```python
from build123d import *

# Parameters (mm, degrees)
SKETCH1_R           = 11.15
BOSS_EXTRUDE1_DEPTH = 50
SKETCH2_R           = 7.75
BOSS_EXTRUDE2_DEPTH = 8
SKETCH3_R           = 5.825
BOSS_EXTRUDE3_DEPTH = 10
SKETCH4_R           = 9.1
CUT_EXTRUDE1_DEPTH  = 35
SKETCH5_R           = 2.75
CUT_EXTRUDE2_DEPTH  = 70.804333676
SKETCH10_W          = 3
SKETCH10_H          = 11.4427922
BOSS_EXTRUDE5_DEPTH = 6
SKETCH12_W          = 6
SKETCH12_H          = 1
CUT_EXTRUDE6_DEPTH  = 6
CUT_EXTRUDE8_DEPTH  = 18
SKETCH14_W          = 6
SKETCH14_H          = 10.4427922
CUT_EXTRUDE9_DEPTH  = 8


with BuildPart() as part:
    # Sketch1 → Boss-Extrude1 (new body)
    with BuildSketch(Plane(origin=(0, 0, 0), x_dir=(1, 0, 0), z_dir=(0, 1, 0))):
        with Locations(Location((0, 0, 0), (0, 0, 270))):
            Circle(SKETCH1_R)
    extrude(amount=BOSS_EXTRUDE1_DEPTH)

    # Sketch2 → Boss-Extrude2 (add)
    with BuildSketch(Plane(origin=(0, 50, 0), x_dir=(1, 0, 0), z_dir=(0, 1, 0))):
        with Locations(Location((0, 0, 0), (0, 0, 270))):
            Circle(SKETCH2_R)
    extrude(amount=BOSS_EXTRUDE2_DEPTH)

    # Sketch3 → Boss-Extrude3 (add)
    with BuildSketch(Plane(origin=(0, 58, 0), x_dir=(1, 0, 0), z_dir=(0, 1, 0))):
        with Locations(Location((0, 0, 0), (0, 0, 270))):
            Circle(SKETCH3_R)
    extrude(amount=BOSS_EXTRUDE3_DEPTH)

    # Sketch4 → Cut-Extrude1 (cut)
    with BuildSketch(Plane.XZ):
        with Locations(Location((0, 0, 0), (0, 0, 270))):
            Circle(SKETCH4_R)
    extrude(amount=-CUT_EXTRUDE1_DEPTH, mode=Mode.SUBTRACT)

    # Sketch5 → Cut-Extrude2 (cut, through all)
    with BuildSketch(Plane(origin=(0, 68, 0), x_dir=(1, 0, 0), z_dir=(0, 1, 0))):
        with Locations(Location((0, 0, 0), (0, 0, 270))):
            Circle(SKETCH5_R)
    extrude(amount=-CUT_EXTRUDE2_DEPTH, mode=Mode.SUBTRACT)


with BuildPart() as body_2:
    # Sketch10 → Boss-Extrude5 (new body)
    with BuildSketch(Plane(origin=(0, 58, 0), x_dir=(1, 0, 0), z_dir=(0, 1, 0))):
        with Locations((-1.5, -13.4713961)):
            Rectangle(SKETCH10_W, SKETCH10_H)
        with Locations((1.5, -13.4713961)):
            Rectangle(SKETCH10_W, SKETCH10_H)
    extrude(amount=-BOSS_EXTRUDE5_DEPTH)

    # Sketch12 → Cut-Extrude6 (cut)
    with BuildSketch(Plane(origin=(0, 58, 0), x_dir=(1, 0, 0), z_dir=(0, 1, 0))):
        with Locations((0, -8.25)):
            Rectangle(SKETCH12_W, SKETCH12_H)
    extrude(amount=-CUT_EXTRUDE6_DEPTH, mode=Mode.SUBTRACT)


with BuildPart() as cut_extrude8_tool:
    # Sketch11 → Cut-Extrude8 (new body)
    with BuildSketch(Plane.XY.offset(19.1927922)):
        with BuildLine():
            ThreePointArc((2.95, 55), (0, 57.95), (-2.95, 55))
            Line((-2.95, 55), (2.95, 55))
        make_face()
        with BuildLine():
            Line((2.95, 55), (-2.95, 55))
            ThreePointArc((-2.95, 55), (0, 52.05), (2.95, 55))
        make_face()
    extrude(amount=-CUT_EXTRUDE8_DEPTH)


with BuildPart() as part_1:
    add(part.part)

    # Cut-Extrude8: cut by cut_extrude8_tool
    add(cut_extrude8_tool.part, mode=Mode.SUBTRACT)


with BuildPart() as body_2_1:
    add(body_2.part)

    # Cut-Extrude8: cut by cut_extrude8_tool
    add(cut_extrude8_tool.part, mode=Mode.SUBTRACT)

    # Sketch14 → Cut-Extrude9 (cut)
    with BuildSketch(Plane(origin=(0, 58, 0), x_dir=(1, 0, 0), z_dir=(0, 1, 0))):
        with Locations((0, -13.9713961)):
            Rectangle(SKETCH14_W, SKETCH14_H)
    extrude(amount=-CUT_EXTRUDE9_DEPTH, mode=Mode.SUBTRACT)


solid = part_1.part
```
Source: CAD feature listing. Evaluate the final solid. Frame: model axes, mm. A direction names the side the tool comes from. Give positions to 0.01 mm unless a question says otherwise; leave off trailing zeros. Loops run counter-clockwise (first coordinate to the right, second up) from the corner with the lowest first, then second, coordinate; pieces in that order, holes last. Notation, with made-up numbers: M 64.5,52 L 99.5,52 A30 cw 99.5,86 Z; hole C -22,-37.75 d9. An arc over 180 degrees is marked long. Put each result on its own line as item: value.
Q1. Section C-C (y = 9). Return the cut outline in (x, z), and give its area (3 significant figures).
Response values:
outline: C 0,0 d22.3; hole C 0,0 d18.2
area: 130 mm²
Q2. Mould query, pull axis Y, two halves, no side actions, for faces 1 (the flat face through (2.1, 35, 2.1)), 2 (the flat face through (8, 50, 2)), 3 (the cylindrical face through (0.384, 52.075, 4.517)). Classes: released by +Y, released by -Y, zero draft, split by the parting line, or undercut.
Response values:
face 1: released by -Y
face 2: released by +Y
face 3: undercut
Q3. Line query: probe 1 along X at (y, z) = (61, 0) (3 decimals); probe 2 along Y at (x, z) = (-4.75, -1.25); probe 3 along Z at (x, y) = (-8.25, 30.5). Output: solid intervals per line, ascending. Write a range as [from, to].
Response values:
probe 1: x = [-5.825, -2.75], [2.75, 5.825]
probe 2: y = [35, 68]
probe 3: z = [-7.5, -3.84], [3.84, 7.5]
Q4. Reachability of faces 4 (the cylindrical face through (-5.54, 17.26, 7.22)), 5 (the cylindrical face through (-5.686, 62.93, -1.263)), 6 (the cylindrical face through (0.121, 51.731, -2.747)) from +Z, -Z, +X, -X, +Y, -Y: full face, straight path, thin tool, end or side. Return the list, or none.
Response values:
face 4: -Y
face 5: +Y
face 6: +Y, -Y
Q5. Section A-A (x = 0). Return the cut outline in (y, z) (3 decimals), and give its area (4 significant figures).
Response values:
outline: M 0,-11.15 L 50,-11.15 L 50,-7.75 L 58,-7.75 L 58,-5.825 L 68,-5.825 L 68,-2.75 L 35,-2.75 L 35,-9.1 L 0,-9.1 Z; M 0,9.1 L 35,9.1 L 35,2.75 L 52.05,2.75 L 52.05,7.75 L 50,7.75 L 50,11.15 L 0,11.15 Z; M 57.95,2.75 L 68,2.75 L 68,5.825 L 58,5.825 L 58,7.75 L 57.95,7.75 Z
area: 507.5 mm²
Q6. Pin query (flat end, axial travel): P1, Ø12, axis at y = 59.5, z = -1.5, coming from the +X side; P2, Ø8, axis at y = 30.5, z = -6, coming from the -X side; P3, Ø10, axis at y = 34.5, z = 5, coming from the -X side; P4, Ø4, axis at x = -2.5, y = 35.5, coming from the +Z side. Return the tip coordinate at first contact, or that it passes through.
Response values:
P1: stops at x = 7.75
P2: stops at x = -10.97
P3: stops at x = -11.15
P4: stops at z = 11.14
Q7. Section D-D (z = 4.5). Return the cut outline in (x, y), and give its area (3 significant figures).
Response values:
outline: M -10.2,0 L -7.91,0 L -7.91,35 L 7.91,35 L 7.91,0 L 10.2,0 L 10.2,50 L 6.31,50 L 6.31,58 L 3.7,58 L 3.7,68 L -3.7,68 L -3.7,58 L -6.31,58 L -6.31,50 L -10.2,50 Z; hole C 0,55 d5.9
area: 614 mm²
Q8. Section B-B (z = 0). Return the cut outline in (x, y) (3 decimals).
Response values:
outline: M -11.15,0 L -9.1,0 L -9.1,35 L -2.75,35 L -2.75,68 L -5.825,68 L -5.825,58 L -7.75,58 L -7.75,50 L -11.15,50 Z; M 2.75,35 L 9.1,35 L 9.1,0 L 11.15,0 L 11.15,50 L 7.75,50 L 7.75,58 L 5.825,58 L 5.825,68 L 2.75,68 Z
